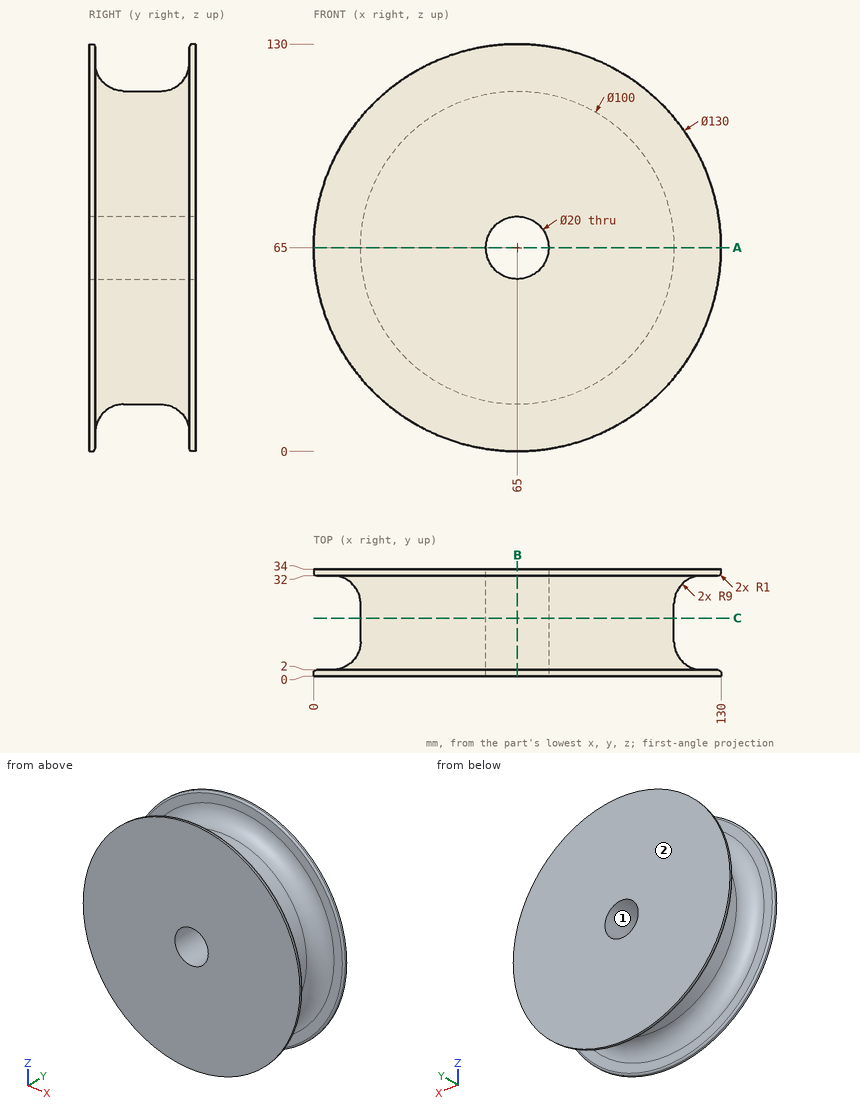
Print and shaded views of the part. All mm, measured from the part's lowest x, y and z. Round coordinates to 2 decimals unless told otherwise and drop trailing zeros. Write each loop counter-clockwise with the first axis right and the second up, starting at its lowest first coordinate (ties: lowest second). Pieces come first, ordered by that corner, then holes. Notation, with made-up numbers: M 66.5,75.25 L 124.5,75.25 A27 cw 124.5,100.25 Z; hole C 33.5,19 d2. An arc over 180 degrees is marked long. Use a Markdown table: item, result. Add a question column.
1. Slice it at C-C on y = 18.5. Give the cut face in (x, z).
2. Slice it at A-A on z = 65. Give the cut face in (x, y).
3. Slice it at B-B on x = 65. Give the cut face in (y, z), then the cut area to 3 significant figures.
4. Pull direction Z, two halves, no side cores. Call the marked faces 1 and 2: released by +Z, released by -Z, zero draft, split by the parting line, or undercut.
5. Flat gauge pins, fed straight in: P1, Ø10, axis at y = 18, z = 15.5, coming from the +X side; P2, Ø6, axis at y = 26, z = 64.5, coming from the -X side; P3, Ø5, axis at x = 59.5, y = 24.5, coming from the +Z side. Where does each tip first touch, or does it go through?
6. Drill centre lines: probe 1 along Z at (x, y) = (65, 23); probe 2 along Y at (x, z) = (19.5, 108.5). Where is each one in solid material? Low to high.
Reply:
| question | item | result |
|---|---|---|
| 1 | outline | C 65,65 d100; hole C 65,65 d20 |
| 2 | outline | M 0,0 L 55,0 L 55,34 L 0,34 L 0,33 A1 ccw 1,32 L 6,32 A9 cw 15,23 L 15,11 A9 cw 6,2 L 1,2 A1 ccw 0,1 Z; M 75,0 L 130,0 L 130,1 A1 ccw 129,2 L 124,2 A9 cw 115,11 L 115,23 A9 cw 124,32 L 129,32 A1 ccw 130,33 L 130,34 L 75,34 Z |
| 3 | outline | M 0,0 L 1,0 A1 ccw 2,1 L 2,6 A9 cw 11,15 L 23,15 A9 cw 32,6 L 32,1 A1 ccw 33,0 L 34,0 L 34,55 L 0,55 Z; M 0,75 L 34,75 L 34,130 L 33,130 A1 ccw 32,129 L 32,124 A9 cw 23,115 L 11,115 A9 cw 2,124 L 2,129 A1 ccw 1,130 L 0,130 Z |
| 3 | area | 2,910 mm^2 |
| 4 | face 1 | undercut |
| 4 | face 2 | zero draft |
| 5 | P1 | stops at x = 87.8 |
| 5 | P2 | stops at x = 12.71 |
| 5 | P3 | stops at z = 115.67 |
| 6 | probe 1 | z = 15 to 55, 75 to 115 |
| 6 | probe 2 | y = 0 to 2, 32 to 34 |
